Answer from the drawing. Dimensions are ordinates in mm from the lowest x, y and z of the part. A direction names the side the tool comes from. Round coordinates to 2 decimals unless told otherwise and drop trailing zeros. Write each loop counter-clockwise with the first axis right and the second up, starting at its lowest first coordinate (ties: lowest second). Pieces come first, ordered by that corner, then holes. Notation, with made-up numbers: (-2.5, 61) - (1.5, 61) arc R20 ccw to (1.5, 86) - close; hole circle Ø7 at (30, -5.75). An arc over 180 degrees is marked (long way). Answer as a JSON object with one key per item and string values.
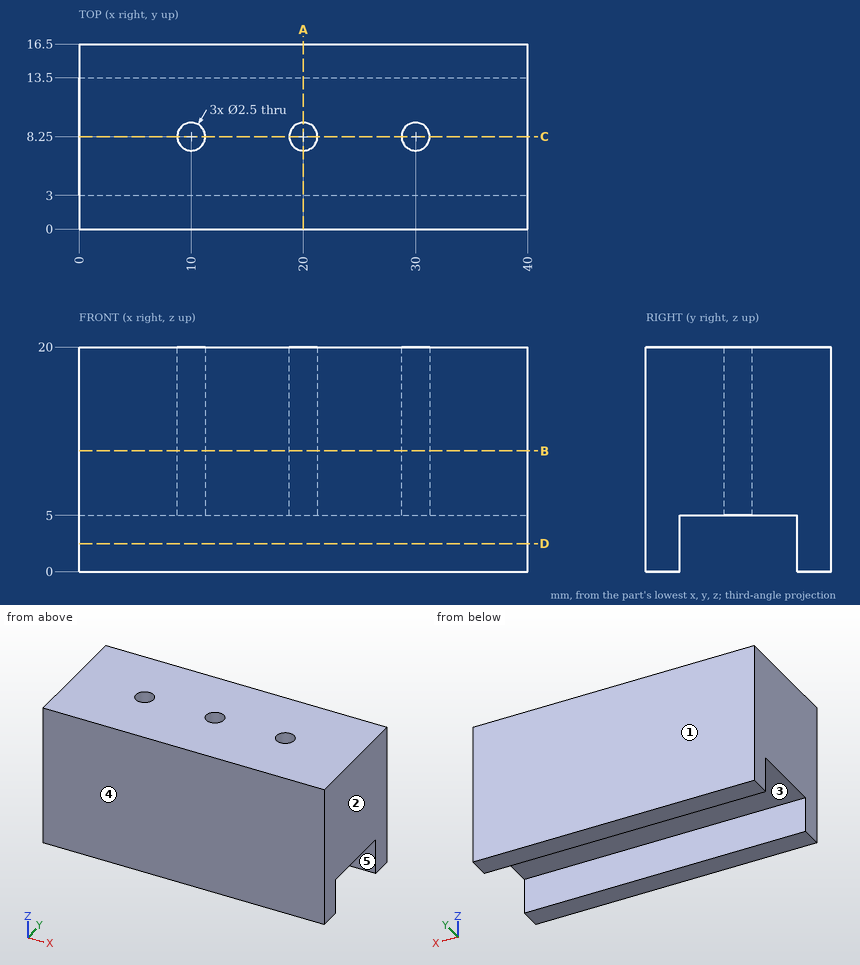
Item 1: A cutting plane is placed at B-B (z = 10.75). Write down the section's boundary in (x, y), and give its area (3 significant figures).
Results found:
{"outline": "(0, 0) - (40, 0) - (40, 16.5) - (0, 16.5) - close; hole circle Ø2.5 at (10, 8.25); hole circle Ø2.5 at (20, 8.25); hole circle Ø2.5 at (30, 8.25)", "area": "645 mm²"}
Item 2: Consider line 1 along Y through (x, z) = (20.5, 1.5); line 2 along Y through (x, z) = (10, 10); line 3 along Z through (x, y) = (19, 11). Determine where each line is inside the solid, lowest interval first.
Results found:
{"line 1": "0 to 3, 13.5 to 16.5", "line 2": "0 to 7, 9.5 to 16.5", "line 3": "5 to 20"}
Item 3: A cutting plane is placed at D-D (z = 2.5). Write down the section's boundary in (x, y), and give its area (3 significant figures).
Results found:
{"outline": "(0, 0) - (40, 0) - (40, 3) - (0, 3) - close; (0, 13.5) - (40, 13.5) - (40, 16.5) - (0, 16.5) - close", "area": "240 mm²"}
Item 4: A cutting plane is placed at A-A (x = 20). Write down the section's boundary in (y, z).
Results found:
{"outline": "(0, 0) - (3, 0) - (3, 5) - (7, 5) - (7, 20) - (0, 20) - close; (9.5, 5) - (13.5, 5) - (13.5, 0) - (16.5, 0) - (16.5, 20) - (9.5, 20) - close"}
Item 5: Determine the mould class of the marked faces 1, 2 and 3 for opening direction Y: pulls with the +Y half, pulls with the -Y half, needs draft (parallel to the pull), parting line crosses it, or undercut.
Results found:
{"face 1": "pulls with the +Y half", "face 2": "needs draft", "face 3": "undercut"}
Item 6: A cutting plane is placed at C-C (y = 8.25). Write down the section's boundary in (x, z).
Results found:
{"outline": "(0, 5) - (8.75, 5) - (8.75, 20) - (0, 20) - close; (11.25, 5) - (18.75, 5) - (18.75, 20) - (11.25, 20) - close; (21.25, 5) - (28.75, 5) - (28.75, 20) - (21.25, 20) - close; (31.25, 5) - (40, 5) - (40, 20) - (31.25, 20) - close"}
Item 7: For the marked faces 4 and 5, determine the directions among +Z, -Z, +X, -X, +Y, -Y from which every point of the face is accessible in a straight line to the end or side of a thin tool.
Results found:
{"face 4": "+Z, -Z, +X, -X, -Y", "face 5": "-Z, +X, -X"}
Item 8: Each of these flat-tipped pins is pushed along its axis until it touches: P1, Ø1.5, axis at x = 13, z = 1.5, coming from the -Y side; P2, Ø3, axis at x = 27, y = 8, coming from the -Z side; P3, Ø2, axis at x = 20, y = 8.25, coming from the +Z side. Where does it stop, or does it pass through?
Results found:
{"P1": "y = 0", "P2": "z = 5", "P3": "through"}
